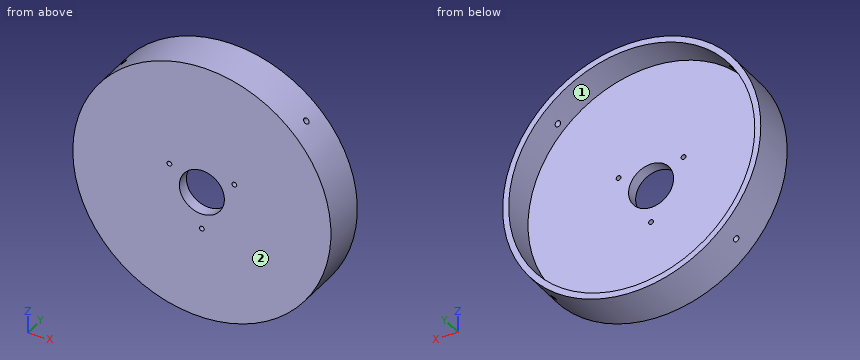
from build123d import *

# Parameters (mm, degrees)
SKETCH2_R          = 0.8
CUT_EXTRUDE1_DEPTH = 62.798058222
SKETCH3_R          = 1
CUT_EXTRUDE2_DEPTH = 63.633856659
CIRPATTERN1_COUNT  = 4


with BuildPart() as part:
    # Sketch1 → Revolve1 (revolve)
    with BuildSketch(Plane.XY, mode=Mode.PRIVATE) as revolve1_sk:
        Polygon((7.5, 4), (7.5, 0), (43, 0), (43, 15), (41, 15), (41, 4), align=None)
    revolve(revolve1_sk.sketch.rotate(Axis((0, 4, 0), (0, -1, 0)), 180), axis=Axis((0, 4, 0), (0, -1, 0)))

    # Sketch2 → Cut-Extrude1 (cut, through all)
    with BuildSketch(Plane(origin=(0, 4, 0), x_dir=(1, 0, 0), z_dir=(0, 1, 0))):
        with Locations(Location((0, 12.5, 0), (0, 0, 180))):
            Circle(SKETCH2_R)
        with Locations(Location((10.825317547, -6.25, 0), (0, 0, 180))):
            Circle(SKETCH2_R)
        with Locations(Location((-10.825317547, -6.25, 0), (0, 0, 180))):
            Circle(SKETCH2_R)
    extrude(amount=-CUT_EXTRUDE1_DEPTH, mode=Mode.SUBTRACT)

    # Sketch3 → Cut-Extrude2 (cut, through all)
    with BuildSketch(Plane(origin=(0, 0, 0), x_dir=(0.7071067811865464, 0, 0.7071067811865488), z_dir=(-0.7071067811865488, 0, 0.7071067811865464))):
        with Locations((0, 7.5)):
            Circle(SKETCH3_R)
    cut_extrude2 = extrude(amount=-CUT_EXTRUDE2_DEPTH, mode=Mode.SUBTRACT)

    # CirPattern1: Cut-Extrude2 ×4 about axis
    cirpattern1_axis = Axis((0, 4, 0), (0, 1, 0))
    for i in range(1, CIRPATTERN1_COUNT):
        add(cut_extrude2.rotate(cirpattern1_axis, i * 360 / CIRPATTERN1_COUNT), mode=Mode.SUBTRACT)


solid = part.part
Check sheet for the modelled part. Datum: model origin and axes. Units: mm. Face numbers are marked on the shaded views. A direction names the side the tool comes from. Round coordinates to 2 decimals unless told otherwise and drop trailing zeros. Write each loop counter-clockwise with the first axis right and the second up, starting at its lowest first coordinate (ties: lowest second). Pieces come first, ordered by that corner, then holes. Notation, with made-up numbers: (-30.75, -2) - (-11.75, -2) arc R18 cw to (-11.75, 13) - close; hole circle Ø5 at (-10.5, 50.25). An arc over 180 degrees is marked (long way). Return JSON: item names as keys, results as strings.
Q1. Cross-section at D-D (z = -18). Record the boundary of the cut face in (x, y), then the cut area to 3 significant figures.
Returned:
{"outline": "(-39.05, 0) - (39.05, 0) - (39.05, 15) - (36.84, 15) - (36.84, 4) - (-36.84, 4) - (-36.84, 15) - (-39.05, 15) - close", "area": "361 mm²"}
Q2. Cross-section at B-B (x = 6). Record the boundary of the cut face in (y, z).
Returned:
{"outline": "(0, -42.58) - (15, -42.58) - (15, -40.56) - (4, -40.56) - (4, -4.5) - (0, -4.5) - close; (0, 4.5) - (4, 4.5) - (4, 40.56) - (15, 40.56) - (15, 42.58) - (0, 42.58) - close"}
Q3. Scan lines: L1, parallel to Z at x = 0, y = 2.75; L2, parallel to Z at x = 1, y = 7.25; L3, parallel to Y at x = 13, z = -26.5. Record each from-to range of solid material in increasing order. Write a range as from..to.
Returned:
{"L1": "z = -43..-13.3, -11.7..-7.5, 7.5..43", "L2": "z = -42.99..-40.99, 40.99..42.99", "L3": "y = 0..4"}
Q4. Access from +Z, -Z, +X, -X, +Y, -Y to the whole of each face (thin tool, end or side, straight path). Record for the marked faces 1 and 2.
Returned:
{"face 1": "+Y", "face 2": "+Z, -Z, +X, -X, -Y"}
Q5. Cross-section at A-A (z = 0). Record the boundary of the cut face in (x, y), then the cut area to 3 significant figures.
Returned:
{"outline": "(-43, 0) - (-7.5, 0) - (-7.5, 4) - (-41, 4) - (-41, 15) - (-43, 15) - close; (7.5, 0) - (43, 0) - (43, 15) - (41, 15) - (41, 4) - (7.5, 4) - close", "area": "328 mm²"}
Q6. Depth check by flat-ended pin: P1, Ø8, axis at x = -34, y = 10.5, coming from the -Z side; P2, Ø6, axis at y = 12, z = -12.5, coming from the +X side; P3, Ø24.5, axis at x = 3.5, z = -19, coming from the +Y side. Enter the tip coordinate at first touch or a pass-through.
Returned:
{"P1": "stops at z = -30.81", "P2": "stops at x = 41.94", "P3": "stops at y = 4"}
Q7. Cross-section at C-C (y = 2.75). Record the boundary of the cut face in (x, z), then the cut area to 3 significant figures.
Returned:
{"outline": "circle Ø86 at (0, 0); hole circle Ø1.6 at (-10.83, 6.25); hole circle Ø15 at (0, 0); hole circle Ø1.6 at (0, -12.5); hole circle Ø1.6 at (10.83, 6.25)", "area": "5,630 mm²"}
